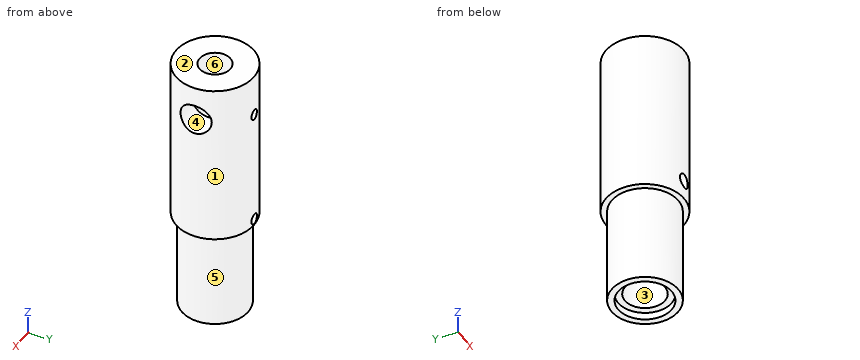
from build123d import *

# Parameters (mm, degrees)
SKETCH1_R          = 10.8204
SKETCH1_R_2        = 8.7122
EXTRUDE1_DEPTH     = 86.36
SKETCH2_R          = 12.7
SKETCH2_R_2        = 2.5908
EXTRUDE2_DEPTH     = 53.975
SKETCH3_R          = 8.7122
SKETCH3_R_2        = 6.5151
EXTRUDE3_DEPTH     = 35.3822
SKETCH4_R          = 8.7122
SKETCH4_R_2        = 6.5151
CUT_EXTRUDE1_DEPTH = 2.3876
SKETCH15_R         = 2.3622
CUT_EXTRUDE5_DEPTH = 7.2644
SKETCH17_R         = 1.7018
CUT_EXTRUDE6_DEPTH = 4.572
SKETCH18_R         = 5.0165
CUT_EXTRUDE7_DEPTH = 8.382
SKETCH19_R         = 5.0165
CUT_EXTRUDE8_DEPTH = 8.382


with BuildPart() as part:
    # Sketch1 → Extrude1 (new body)
    with BuildSketch(Plane.XY):
        Circle(SKETCH1_R)
        Circle(SKETCH1_R_2, mode=Mode.SUBTRACT)
    extrude(amount=EXTRUDE1_DEPTH)

    # Sketch2 → Extrude2 (add)
    with BuildSketch(Plane.XY.offset(86.36)):
        Circle(SKETCH2_R)
        Circle(SKETCH2_R_2, mode=Mode.SUBTRACT)
    extrude(amount=-EXTRUDE2_DEPTH)

    # Sketch3 → Extrude3 (add)
    with BuildSketch(Plane(origin=(0, 0, 0), x_dir=(-1, 0, 0), z_dir=(0, 0, -1))):
        Circle(SKETCH3_R)
        Circle(SKETCH3_R_2, mode=Mode.SUBTRACT)
    extrude(amount=-EXTRUDE3_DEPTH)

    # Sketch4 → Cut-Extrude1 (cut)
    with BuildSketch(Plane(origin=(0, 0, 0), x_dir=(-1, 0, 0), z_dir=(0, 0, -1))):
        Circle(SKETCH4_R)
        Circle(SKETCH4_R_2, mode=Mode.SUBTRACT)
    extrude(amount=-CUT_EXTRUDE1_DEPTH, mode=Mode.SUBTRACT)

    # Sketch15 → Cut-Extrude5 (cut)
    with BuildSketch(Plane(origin=(0, -12.7, 0), x_dir=(-1, 0, 0), z_dir=(0, 1, 0))):
        with Locations(Location((0, 38.8874, 0), (0, 0, 270))):  # turned: the seam where the file's is
            Circle(SKETCH15_R)
    extrude(amount=CUT_EXTRUDE5_DEPTH, mode=Mode.SUBTRACT)

    # Sketch17 → Cut-Extrude6 (cut)
    with BuildSketch(Plane(origin=(0, 12.7, 0), x_dir=(-1, 0, 0), z_dir=(0, 1, 0))):
        with Locations(Location((0, 34.3916, 0), (0, 0, 90))):  # turned: the seam where the file's is
            Circle(SKETCH17_R)
        with Locations(Location((0, 72.4408, 0), (0, 0, 90))):  # turned: the seam where the file's is
            Circle(SKETCH17_R)
    extrude(amount=-CUT_EXTRUDE6_DEPTH, mode=Mode.SUBTRACT)

    # Sketch18 → Cut-Extrude7 (cut)
    with BuildSketch(Plane.XY.offset(86.36)):
        Circle(SKETCH18_R)
    extrude(amount=-CUT_EXTRUDE7_DEPTH, mode=Mode.SUBTRACT)

    # Sketch19 → Cut-Extrude8 (cut)
    with BuildSketch(Plane(origin=(12.7, 0, 0), x_dir=(0, 0, -1), z_dir=(1, 0, 0))):
        with Locations(Location((-74.93, 0, 0), (0, 0, 180))):  # turned: the seam where the file's is
            Circle(SKETCH19_R)
    extrude(amount=-CUT_EXTRUDE8_DEPTH, mode=Mode.SUBTRACT)


solid = part.part
Geometry check sheet. Reference: the model listing, model coordinates, mm. Face numbers are marked on the shaded views. A direction names the side the tool comes from. Give positions to 0.01 mm unless a question says otherwise; leave off trailing zeros. Write each loop counter-clockwise with the first axis right and the second up, starting at its lowest first coordinate (ties: lowest second). Pieces come first, ordered by that corner, then holes. Notation, with made-up numbers: M 51.5,20.5 L 60.5,20.5 A20 ccw 60.5,52.5 Z; hole C 87,10 d11. An arc over 180 degrees is marked long. One line per question, with ' | ' between items.
1. Gauge pin test, flat ends, axial feed: pin 1 (3 mm diameter, centred on x = -1, y = -1.5, fed in from +Z); pin 2 (2.5 mm diameter, centred on x = 0.5, z = 34.5, fed in from +Y); pin 3 (8 mm diameter, centred on x = 4.5, z = 49, fed in from +Y). Record the tip position at first contact, or that the pin passes through.
Ans:
pin 1: z = 77.98 | pin 2: y = 12.62 | pin 3: y = 12.69
2. Cross-section at C-C (x = -7.75). Enter the section's corners in (y, z) (3 decimals).
Ans:
outline: M -10.061,32.385 L -7.551,32.385 L -7.551,0 L -3.98,0 L -3.98,2.388 L 3.98,2.388 L 3.98,0 L 7.551,0 L 7.551,32.385 L 10.061,32.385 L 10.061,86.36 L -10.061,86.36 Z
3. Mould release check, pull along X, two halves, no side actions. Record for the marked faces 1, 2 and 3: released by +X, released by -X, zero draft, split by the parting line, or undercut.
Ans:
face 1: split by the parting line | face 2: zero draft | face 3: undercut
4. Cross-section at B-B (z = 48.5). Enter the section's corners in (x, y), plus the area to 3 significant figures.
Ans:
outline: C 0,0 d25.4; hole C 0,0 d5.18 | area: 486 mm2
5. Set-up check for the marked faces 4, 5 and 6: record each of +Z, -Z, +X, -X, +Y, -Y from which the full face is reachable in a straight line by a thin tool's end or side.
Ans:
face 4: +X | face 5: -Z | face 6: +Z
6. Scan lines: line 1 along Z through (x, y) = (0, 11.8) (3 decimals); line 2 along Z through (x, y) = (0, 10.3); line 3 along Y through (x, z) = (0, 1.6). Record each from-to range of solid material in increasing order. Write a range as from..to.
Ans:
line 1: 32.385..32.69, 36.093..70.739, 74.143..86.36 | line 2: 0..32.69, 36.09..70.74, 74.14..86.36 | line 3: -10.82..-8.71, 8.71..10.82
7. Cross-section at D-D (x = -4.25). Enter the section's corners in (y, z) (3 decimals).
Ans:
outline: M -11.968,32.385 L -9.951,32.385 L -9.951,0 L -7.605,0 L -7.605,2.388 L -4.938,2.388 L -4.938,32.385 L 4.938,32.385 L 4.938,2.388 L 7.605,2.388 L 7.605,0 L 9.951,0 L 9.951,32.385 L 11.968,32.385 L 11.968,86.36 L 2.665,86.36 L 2.665,77.978 L -2.665,77.978 L -2.665,86.36 L -11.968,86.36 Z
8. Cross-section at A-A (y = 0). Enter the section's corners in (x, z) (1 decimal).
Ans:
outline: M -12.7,32.4 L -10.8,32.4 L -10.8,0 L -8.7,0 L -8.7,2.4 L -6.5,2.4 L -6.5,32.4 L -2.6,32.4 L -2.6,78 L -5,78 L -5,86.4 L -12.7,86.4 Z; M 2.6,32.4 L 6.5,32.4 L 6.5,2.4 L 8.7,2.4 L 8.7,0 L 10.8,0 L 10.8,32.4 L 12.7,32.4 L 12.7,69.9 L 4.3,69.9 L 4.3,78 L 2.6,78 Z; M 5,79.9 L 12.7,79.9 L 12.7,86.4 L 5,86.4 Z
